Autodesk Inventor part; units mm, degrees
ref_plane "YZ Plane" through (0, 0, 0) normal (1, 0, 0) x (0, 1, 0)
ref_plane "XZ Plane" through (0, 0, 0) normal (0, 1, 0) x (-1, 0, 0)
ref_plane "XY Plane" through (0, 0, 0) normal (0, 0, 1) x (1, 0, 0)
sketch "Sketch1" plane through (0, 0, 0) normal (0, 0, 1) x (1, 0, 0)
  line L0 (-4.5, 11) -> (4.5, 11)
  line L1 (4.5, 11) -> (4.5, 0)
  line L2 (4.5, 0) -> (-4.5, 0)
  line L3 (-4.5, 0) -> (-4.5, 11)
  point P0 (0, 0)
  dimension "d0" = 9
  dimension "d1" = 0
  dimension "d2" = 11
  dimension "d3" = 4.5
extrude "Extrusion1" add sketch "Sketch1" against normal blind 15.3
sketch "Sketch2" plane through (0, 0, 0) normal (0, 0, 1) x (1, 0, 0)
  line L0 (4.5, 0) -> (-4.5, 0)
  circle A0 centre (0, 6.5) radius 2.85
  point P0 (0, 0)
  dimension "d6" = 5.7
  dimension "d7" = 6.5
extrude "Extrusion2" cut sketch "Sketch2" against normal blind 10
sketch "Sketch4" plane through (0, 0, 0) normal (0, 0, 1) x (1, 0, 0)
  circle A0 centre (0, 6.5) radius 2.85
  line L0 (4.5, 11) -> (4.5, 0)
  arc A1 (-3.1623, 8) -> (-3.1623, 5) centre (0, 6.5) ccw
  arc A2 (3.1623, 5) -> (3.1623, 8) centre (0, 6.5) ccw
  line L1 (-3.1623, 8) -> (3.1623, 8)
  line L2 (-3.1623, 5) -> (3.1623, 5)
  point P0 (0, 0)
  dimension "d17" = 3.5
  dimension "d18" = 3
  dimension "d19" = 1.5
extrude "Extrusion4" cut sketch "Sketch4" against normal blind 2 contours A0 L2 L1 | A0 L1 A2 L2 | A0 L2 A1 L1
sketch "Sketch3" plane through (0, 6.5, -10) normal (0, 0, 1) x (1, 0, 0)
  circle A0 centre (0, 0) radius 2.85
  circle A1 centre (0, 0) radius 1.25
  point P0 (0, -6.5)
  dimension "d10" = 2.5
extrude "Extrusion3" add sketch "Sketch3" along normal blind 9 contours A1
fillet "Fillet1" radius 1.25 1 edges at (-1.25, 6.5, -1)
sketch "Sketch5" plane through (0, 0, -15.3) normal (0, 0, -1) x (-1, 0, 0)
  line L0 (4.5, 11) -> (-4.5, 11)
  line L1 (-4.5, 11) -> (-4.5, 0)
  line L2 (-4.5, 0) -> (4.5, 0)
  line L3 (4.5, 0) -> (4.5, 11)
  arc A0 (4.5, 6.5) -> (-4.5, 6.5) centre (0, 6.5) ccw
  point P0 (0, 0)
  dimension "d22" = 0
  dimension "d23" = 9
extrude "Extrusion5" cut sketch "Sketch5" against normal blind 12.3 contours L3 A0 L0 | A0 L1 L0
properties part number "jack" material "PET Plastic"
CAD build for the part. Positions are in the model's coordinates, mm. A direction names the side the tool comes from. Round coordinates to 2 decimals unless told otherwise and drop trailing zeros. Write each loop counter-clockwise with the first axis right and the second up, starting at its lowest first coordinate (ties: lowest second). Pieces come first, ordered by that corner, then holes. Notation, with made-up numbers: M 81.5,43.5 L 102.5,43.5 A20 ccw 102.5,70.5 Z; hole C 17.25,44.25 d10. An arc over 180 degrees is marked long. One line per question, with ' | ' between items.
1. Cut at A-A on z = -1.5. Write the cut outline in (x, y), and give its area (3 significant figures).
Working result:
outline: M -4.5,0 L 4.5,0 L 4.5,11 L -4.5,11 Z; C 0,6.5 d2; hole M -3.16,5 L -2.42,5 A2.85 ccw 2.42,5 L 3.16,5 A3.5 ccw 3.16,8 L 2.42,8 A2.85 ccw -2.42,8 L -3.16,8 A3.5 ccw Z | area: 72.6 mm2
2. Mould opens along Y. For faces 6 (the cylindrical face through (0, 11, -9)), 7 (the flat face through (1, 5, -10)), 8 (the flat face through (0, 3, 0)) say: pulls with the +Y half, pulls with the -Y half, needs draft (parallel to the pull), parting line crosses it, or undercut.
Working result:
face 6: pulls with the +Y half | face 7: undercut | face 8: needs draft
3. Cut at B-B on z = -6.5. Write the cut outline in (x, y), and give its area (3 significant figures).
Working result:
outline: M -4.5,0 L 4.5,0 L 4.5,6.5 A4.5 ccw -4.5,6.5 Z; C 0,6.5 d2.5; hole C 0,6.5 d5.7 | area: 69.7 mm2
4. Which spindle directions (+Z, -Z, +X, -X, +Y, -Y) get a long thin tool onto all of the face, cutting with end or side? Do faces 1 (the flat face through (4.5, 4, -6)), 2 (the flat face through (4, 10, -3)), 3 (the cylindrical face through (-2.847, 6.625, -4.93)), 4 (the flat face through (-3.4, 10.1, -3)), 5 (the flat face through (0, 0, -8)). Say none if no direction does.
Working result:
face 1: +Z, -Z, +X, +Y, -Y | face 2: -Z, +X, +Y | face 3: +Z | face 4: -Z, -X, +Y | face 5: +Z, -Z, +X, -X, -Y
5. Probe L1, parallel to Y at x = 0, z = -6.5; L2, parallel to Y at x = 2.5, z = -0.75; L3, parallel to Y at x = -0.5, z = -6.25. List the from-to ranges inside material, lowest first. Write a range as from..to.
Working result:
L1: 0..3.65, 5.25..7.75, 9.35..11 | L2: 0..5, 8..11 | L3: 0..3.69, 5.35..7.65, 9.31..10.97
6. Cut at D-D on x = -1.5. Write the cut outline in (y, z).
Working result:
outline: M 0,-15.3 L 10.74,-15.3 L 10.74,-3 L 11,-3 L 11,0 L 8.92,0 L 8.92,-10 L 4.08,-10 L 4.08,0 L 0,0 Z
7. Cut at C-C on y = 7.25. Write the cut outline in (x, z).
Working result:
outline: M -4.5,-3 L -4.44,-3 L -4.44,-15.3 L 4.44,-15.3 L 4.44,-3 L 4.5,-3 L 4.5,0 L 3.42,0 L 3.42,-2 L 2.75,-2 L 2.75,-10 L 1,-10 L 1,-2.25 A1 ccw -1,-2.25 L -1,-10 L -2.75,-10 L -2.75,-2 L -3.42,-2 L -3.42,0 L -4.5,0 Z
8. Pin check, flat tips, straight feed: pin 1 Ø0.5 at (x, y) = (3, 7) entering from +Z; pin 2 Ø1.7 at (x, y) = (1.5, 6) entering from +Z; pin 3 Ø2 at (y, z) = (9.5, -9) entering from -X. Stop position of each tip, or through.
Working result:
pin 1: z = -2 | pin 2: z = -1.24 | pin 3: x = -4.03
